Verification items for the finished model (mm, model axes). Face numbers are marked on the shaded views. Coordinates: 2 decimals unless noted, no trailing zeros. Loops run counter-clockwise (first coordinate to the right, second up) from the corner with the lowest first, then second, coordinate; pieces in that order, holes last.
Q1. Sectioned sample at D-D (z = -14.5). Enter the section's corners in (x, y).
Q2. Go/stop test with flat-tipped pins: P1, Ø5, axis at x = 0.5, y = -1.5, coming from the +Z side; P2, Ø3, axis at x = -2, z = -3, coming from the +Y side; P3, Ø1, axis at x = 1.5, z = -7.5, coming from the -Y side. Record where each tip stops, or that it passes through.
Q3. Sectioned sample at A-A (y = 0). Enter the section's corners in (x, z).
Q4. Mould release check, pull along Y, two halves, no side actions. Record for the marked faces 1, 2 and 3: +Y half, -Y half, draft (parallel to the pull), parting line (faces both ways), or undercut.
Q5. Material ranges on probe 1 along Y at (x, z) = (0, -6.5); probe 2 along X at (y, z) = (3, -4.75); probe 3 along Y at (x, z) = (-3.5, -1.75), recorded low to high.
Q6. Sectioned sample at C-C (z = -5.75). Enter the section's corners in (x, y).
```python
from build123d import *

# Parameters (mm, degrees)
SKETCH2_R          = 4.5
CUT_EXTRUDE1_DEPTH = 11
CHAMFER2_SIZE      = 2


with BuildPart() as part:
    # Sketch1 → Revolve1 (revolve)
    with BuildSketch(Plane(origin=(0, 0, 0), x_dir=(0, 0, -1), z_dir=(1, 0, 0)), mode=Mode.PRIVATE) as revolve1_sk:
        Polygon((16.85, -5), (18.1, -5), (18.1, 0), (0, 0), (0, -5), (16.84, -5), (16.84, -4), (16.85, -4), align=None)
    revolve(revolve1_sk.sketch.rotate(Axis((0, 0, 0), (0, 0, -1)), 270), axis=Axis((0, 0, 0), (0, 0, -1)))

    # Sketch2 → Cut-Extrude1 (cut)
    with BuildSketch(Plane.XY):
        Circle(SKETCH2_R)
    extrude(amount=-CUT_EXTRUDE1_DEPTH, mode=Mode.SUBTRACT)

    # Chamfer2
    # the kernel refuses this chamfer: 2 mm, written as the material it takes off along each edge
    with BuildSketch(Plane(origin=(0, 0, -16.84), x_dir=(1, 0, 0), z_dir=(0, 1, 0))) as chamfer2_piece_1_section:
        Polygon((5 - CHAMFER2_SIZE, 0), (5, -CHAMFER2_SIZE), (5, 0), align=None)
    chamfer2_piece_1 = revolve(axis=Axis((0, 0, -16.84), (0, 0, -1)), mode=Mode.PRIVATE)
    chamfer2_piece_1 = chamfer2_piece_1 - Plane(origin=(0, 0, -15.337254953), x_dir=(1, 0, 0), z_dir=(0, 0, -1)) * Cylinder(4, 20, mode=Mode.PRIVATE)
    add(chamfer2_piece_1, mode=Mode.SUBTRACT)


solid = part.part
```
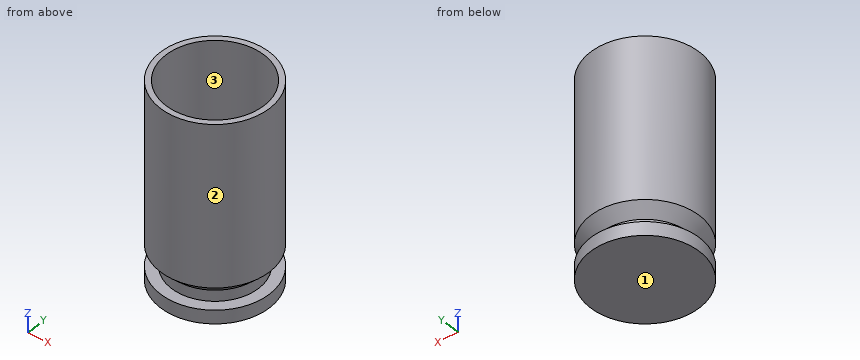
Geometry check:
1. outline: circle Ø10 at (0, 0)
2. P1: stops at z = -11
2. P2: stops at y = 4.97
2. P3: stops at y = -4.9
3. outline: (-5, -18.1) - (5, -18.1) - (5, -16.85) - (4, -16.85) - (4, -15.84) - (5, -14.84) - (5, 0) - (4.5, 0) - (4.5, -11) - (-4.5, -11) - (-4.5, 0) - (-5, 0) - (-5, -14.84) - (-4, -15.84) - (-4, -16.85) - (-5, -16.85) - close
4. face 1: draft
4. face 2: parting line
4. face 3: undercut
5. probe 1: y = -5 to -4.5, 4.5 to 5
5. probe 2: x = -4 to -3.35, 3.35 to 4
5. probe 3: y = -3.57 to -2.83, 2.83 to 3.57
6. outline: circle Ø10 at (0, 0); hole circle Ø9 at (0, 0)
